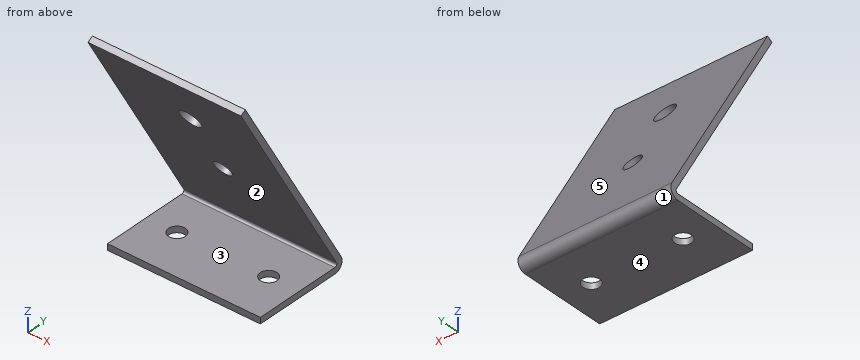
```python
from build123d import *

# Parameters (mm, degrees)
FLANGE_BASE1_DEPTH          = 50
CORTE_EXTRUS_O2_REACH       = 80.784
ESBO_O2_R                   = 3
ESBO_O2_R_2                 = 3.5
FURO_COM_FOLGA_DE_M51_D     = 5.5
FURO_COM_FOLGA_DE_M51_DEPTH = 2


# Sheet-metal steps are written as plain solids
with BuildPart() as part:
    # Esboço1 → Flange-base1 (new body)
    with BuildSketch(Plane(origin=(0, 0, 0), x_dir=(0, 0, -1), z_dir=(1, 0, 0))):
        with BuildLine():
            Line((0, 0), (0, 28.724171375))
            ThreePointArc((0, 28.724171375), (-0.3683, 29.362085688), (-1.1049, 29.362085688))
            Line((-1.1049, 29.362085688), (-64.951905284, -7.5))
            Line((-64.951905284, -7.5), (-65.951905284, -5.767949192))
            Line((-65.951905284, -5.767949192), (-2.1049, 31.094136495))
            ThreePointArc((-2.1049, 31.094136495), (0.6317, 31.094136495), (2, 28.724171375))
            Line((2, 28.724171375), (2, 0))
            Line((2, 0), (0, 0))
        make_face()
    extrude(amount=FLANGE_BASE1_DEPTH)

    # Esboço2 → Corte-extrusão2 (cut, up to next)
    with BuildSketch(Plane(origin=(0, 24.232050808, 13.990381057), x_dir=(1, 0, 0), z_dir=(0, 0.866025403784436, 0.5000000000000044)), mode=Mode.PRIVATE) as corte_extrus_o2_sk1:
        with Locations(Location((25, -15, 0), (0, 0, 270))):
            Circle(ESBO_O2_R)
    corte_extrus_o2_tool1 = extrude(corte_extrus_o2_sk1.sketch, amount=-CORTE_EXTRUS_O2_REACH, mode=Mode.PRIVATE) & part.part
    # Esboço2 → Corte-extrusão2 (cut, up to next)
    with BuildSketch(Plane(origin=(0, 24.232050808, 13.990381057), x_dir=(1, 0, 0), z_dir=(0, 0.866025403784436, 0.5000000000000044)), mode=Mode.PRIVATE) as corte_extrus_o2_sk2:
        with Locations(Location((25, -40, 0), (0, 0, 270))):
            Circle(ESBO_O2_R_2)
    corte_extrus_o2_tool2 = extrude(corte_extrus_o2_sk2.sketch, amount=-CORTE_EXTRUS_O2_REACH, mode=Mode.PRIVATE) & part.part
    add(corte_extrus_o2_tool1.solids().sort_by_distance((25, 16.732051, 26.980762))[0], mode=Mode.SUBTRACT)
    add(corte_extrus_o2_tool2.solids().sort_by_distance((25, 4.232051, 48.631397))[0], mode=Mode.SUBTRACT)

    # Furo com folga de M51
    with Locations(Plane(origin=(0, 0, -2), x_dir=(-1, 0, 0), z_dir=(0, 0, -1))):
        with Locations((-10, 15), (-40, 15)):
            Hole(FURO_COM_FOLGA_DE_M51_D / 2, depth=FURO_COM_FOLGA_DE_M51_DEPTH)


solid = part.part
```
Can you work these out from the model? Positions are in its coordinate system, mm. Face numbers are marked on the shaded views. A direction names the side the tool comes from. Coordinates: 2 decimals unless noted, no trailing zeros. Order: outer loops, then holes, each group sorted by start corner. A loop starts at its lowest first (then second) coordinate and runs counter-clockwise, first axis right, second up. Notation, with made-up numbers: (84, 78) - (109, 78) arc R24 cw to (109, 91) - close; hole circle Ø11 at (77.25, -35). An arc over 180 degrees is marked (long way). Answer in a Markdown table with one row per item.
1. Suppose I cut it at B-B (y = 25). Please give me the cut outline in (x, z).
Reply:
| item | result |
|---|---|
| outline | (0, -2) - (50, -2) - (50, 0) - (0, 0) - close; (0, 8.66) - (50, 8.66) - (50, 12.66) - (0, 12.66) - close |
2. If we mould it in two halves opening along Z, with no side actions, what happens to the marked faces 3, 4 and 5? For each: pulls with the +Z half, pulls with the -Z half, needs draft (parallel to the pull), parting line crosses it, or undercut.
Reply:
| item | result |
|---|---|
| face 3 | undercut |
| face 4 | pulls with the -Z half |
| face 5 | pulls with the +Z half |
3. Suppose I cut it at C-C (x = 23). Please give me the cut outline in (y, z).
Reply:
| item | result |
|---|---|
| outline | (-7.5, 64.95) - (1.06, 50.12) - (2.8, 51.12) - (-5.77, 65.95) - close; (0, -2) - (28.72, -2) arc R2.74 ccw to (31.09, 2.1) - (17.85, 25.04) - (16.12, 24.04) - (29.36, 1.1) arc R0.74 cw to (28.72, 0) - (0, 0) - close; (3.94, 45.14) - (13.88, 27.92) - (15.61, 28.92) - (5.67, 46.14) - close |
4. For the marked faces 1 and 2, which set-ups out of +Z, -Z, +X, -X, +Y, -Y let a thin tool reach every point of the face, with its end or its side?
Reply:
| item | result |
|---|---|
| face 1 | +X, -X, +Y |
| face 2 | +X, -X, -Y |
5. Suppose I cut it at A-A (x = 10). Please give me the cut outline in (y, z).
Reply:
| item | result |
|---|---|
| outline | (-7.5, 64.95) - (29.36, 1.1) arc R0.74 cw to (28.72, 0) - (17.75, 0) - (17.75, -2) - (28.72, -2) arc R2.74 ccw to (31.09, 2.1) - (-5.77, 65.95) - close; (0, -2) - (12.25, -2) - (12.25, 0) - (0, 0) - close |
6. If I drill on line 1 along Z through (x, y) = (27.5, 20.5); line 2 along Y through (x, z) = (10, -1.4); line 3 along Y through (x, z) = (40, -1), over which ranges is the centre line in solid material (lowest first)?
Reply:
| item | result |
|---|---|
| line 1 | z = -2 to 0, 16.45 to 20.45 |
| line 2 | y = 0 to 12.25, 17.75 to 30.43 |
| line 3 | y = 0 to 12.25, 17.75 to 30.84 |
7. For pin 1 (1.5 mm diameter, centred on x = 35.5, z = 46.5, fed in from -Y); pin 2 (2 mm diameter, centred on x = 18.5, z = 8, fed in from -Y); pin 3 (2 mm diameter, centred on x = 45, z = 19, fed in from -Y), each with a flat end and sliding along its axis, tell me the tip position at first contact or that it passes through.
Reply:
| item | result |
|---|---|
| pin 1 | stops at y = 2.72 |
| pin 2 | stops at y = 24.8 |
| pin 3 | stops at y = 18.45 |
8. Suppose I cut it at D-D (x = 36). Please give me the cut outline in (y, z), and give its area (3 significant figures).
Reply:
| item | result |
|---|---|
| outline | (-7.5, 64.95) - (29.36, 1.1) arc R0.74 cw to (28.72, 0) - (0, 0) - (0, -2) - (28.72, -2) arc R2.74 ccw to (31.09, 2.1) - (-5.77, 65.95) - close |
| area | 212 mm^2 |
